```python
from build123d import *

# Parameters (mm, degrees)
F1_R     = 50
F1_R_2   = 40
F3_DEPTH = 25
F2_R     = 50.8307141885
F2_R_2   = 38.5941106118
F2_R_3   = 3.4704975252
F4_DEPTH = 25


with BuildPart() as f3:
    # F1 (on face) → F3 (new body, symmetric)
    with BuildSketch(Plane.XY):
        Circle(F1_R)
        Circle(F1_R_2, mode=Mode.SUBTRACT)
        Circle(F1_R_2)
    extrude(amount=F3_DEPTH, both=True)

    # F2 (on Front) → F4 (join, symmetric)
    with BuildSketch(Plane.XZ):
        Circle(F2_R)
        Circle(F2_R_2, mode=Mode.SUBTRACT)
        Circle(F2_R_2)
        Circle(F2_R_3, mode=Mode.SUBTRACT)
    extrude(amount=F4_DEPTH, both=True)


solid = f3.part
```
Source: CAD feature listing. Evaluate the final solid. Frame: model axes, mm. A direction names the side the tool comes from. Round coordinates to 2 decimals unless told otherwise and drop trailing zeros. Loops run counter-clockwise (first coordinate to the right, second up) from the corner with the lowest first, then second, coordinate; pieces in that order, holes last.
(1) Section query B-B (z = 0). Output: boundary loops of the cut face in (x, y), and give its area (3 significant figures).
From the geometry:
outline: (-50.83, -25) - (-43.3, -25) arc R50 ccw to (43.3, -25) - (50.83, -25) - (50.83, 25) - (43.3, 25) arc R50 ccw to (-43.3, 25) - (-50.83, 25) - close
area: 8,150 mm2
(2) Section query D-D (y = 40). Output: boundary loops of the cut face in (x, z).
From the geometry:
outline: (-30, -25) - (30, -25) - (30, 25) - (-30, 25) - close
(3) Contact query for flat-ended pins moving along their axis: pin 1 Ø7.5 at (x, y) = (-7, 36) entering from -Z; pin 2 Ø1.5 at (x, z) = (11, -9) entering from +Y; pin 3 Ø3 at (x, z) = (40.5, -5) entering from -Y. Output: stop coordinate, or through.
From the geometry:
pin 1: stops at z = -25
pin 2: stops at y = 48.94
pin 3: stops at y = -31.29
(4) Access query for faces 1 (the flat face through (-47, 0, 25)), 2 (the flat face through (-1, 35, 25)), 3 (the cylindrical face through (-50, 0, -19)). Directions: +Z, -Z, +X, -X, +Y, -Y. A direction counts if a zero-diameter tool reaches every point of the face in a straight line with its end or side. Return the directions, or none.
From the geometry:
face 1: +Z, -X, +Y, -Y
face 2: +Z, +X, -X, +Y
face 3: -Z, -X
(5) Pull-direction query (X, two-part tool) for faces 4 (the cylindrical face through (-50, 0, 19)), 5 (the cylindrical face through (50, 0, 19)), 6 (the cylindrical face through (-50.78, -0.35, 2.23)); classes: +X half, -X half, draft (parallel to the pull), parting line (faces both ways), or undercut.
From the geometry:
face 4: -X half
face 5: +X half
face 6: parting line
(6) Section query C-C (y = -10.5). Output: boundary loops of the cut face in (x, z).
From the geometry:
outline: (-48.89, -25) - (-44.26, -25) arc R50.83 ccw to (44.26, -25) - (48.89, -25) - (48.89, -13.93) arc R50.83 ccw to (48.89, 13.93) - (48.89, 25) - (44.26, 25) arc R50.83 ccw to (-44.26, 25) - (-48.89, 25) - (-48.89, 13.93) arc R50.83 ccw to (-48.89, -13.93) - close
(7) Material intervals for probe 1 along Z at (x, y) = (5, 38); probe 2 along Y at (x, z) = (28, -11), sorted ascending.
From the geometry:
probe 1: z = -25 to 25
probe 2: y = -41.42 to 41.42
(8) Section query A-A (x = 0). Output: boundary loops of the cut face in (y, z).
From the geometry:
outline: (-50, -25) - (-25, -25) - (-25, -50.83) - (25, -50.83) - (25, -25) - (50, -25) - (50, 25) - (25, 25) - (25, 50.83) - (-25, 50.83) - (-25, 25) - (-50, 25) - close
